from build123d import *

# Parameters (mm, degrees)
ESQUISSE1_W        = 176
ESQUISSE1_H        = 316
ESQUISSE1_W_2      = 70
ESQUISSE1_H_2      = 110
BOSS_EXTRU_1_DEPTH = 2
CONG_1_R           = 20


with BuildPart() as part:
    # Esquisse1 → Boss.-Extru.1 (new body)
    with BuildSketch(Plane.XY):
        with Locations((88, 158)):
            Rectangle(ESQUISSE1_W, ESQUISSE1_H)
        with Locations((131, 80)):
            Rectangle(ESQUISSE1_W_2, ESQUISSE1_H_2, mode=Mode.SUBTRACT)
    extrude(amount=BOSS_EXTRU_1_DEPTH)

    # Congé1
    cong_1_edges = [part.edges().sort_by_distance(p)[0] for p in [
        (166, 25, 1),
        (166, 135, 1),
        (96, 135, 1),
        (96, 25, 1),
    ]]
    fillet(cong_1_edges, radius=CONG_1_R)


solid = part.part
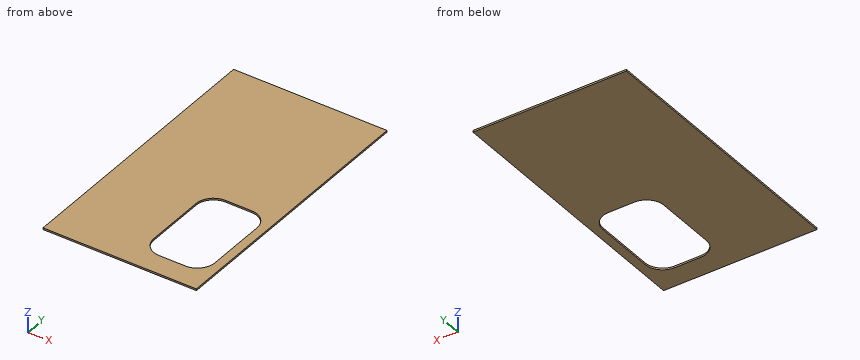
Input: part model. Units: mm. Frame: model coordinates. Coordinates: 2 decimals unless noted, no trailing zeros. Order: outer loops, then holes, each group sorted by start corner. A loop starts at its lowest first (then second) coordinate and runs counter-clockwise, first axis right, second up. Notation, with made-up numbers: M 40.25,59 L 69.25,59 A30 ccw 69.25,97 Z; hole C -36,1.5 d2. An arc over 180 degrees is marked long. Answer in a Markdown table with one row per item.
(1) Section query B-B, the plane z = 0.3. Output: boundary loops of the cut face in (x, y), plus the area to 3 significant figures.
Numbers:
| item | result |
|---|---|
| outline | M 0,0 L 176,0 L 176,316 L 0,316 Z; hole M 96,45 A20 ccw 116,25 L 146,25 A20 ccw 166,45 L 166,115 A20 ccw 146,135 L 116,135 A20 ccw 96,115 Z |
| area | 48,300 mm^2 |
(2) Material intervals for line 1 (X direction, y = 64.5, z = 0.95); line 2 (Y direction, x = 103, z = 1.9); line 3 (Y direction, x = 105.5, z = 0.4), sorted ascending. Write a range as [from, to].
Numbers:
| item | result |
|---|---|
| line 1 | x = [0, 96], [166, 176] |
| line 2 | y = [0, 29.8], [130.2, 316] |
| line 3 | y = [0, 27.98], [132.02, 316] |
(3) Section query C-C, the plane y = 104.5. Output: boundary loops of the cut face in (x, z).
Numbers:
| item | result |
|---|---|
| outline | M 0,0 L 96,0 L 96,2 L 0,2 Z; M 166,0 L 176,0 L 176,2 L 166,2 Z |
(4) Section query A-A, the plane y = 29. Output: boundary loops of the cut face in (x, z), plus the area to 3 significant figures.
Numbers:
| item | result |
|---|---|
| outline | M 0,0 L 104,0 L 104,2 L 0,2 Z; M 158,0 L 176,0 L 176,2 L 158,2 Z |
| area | 244 mm^2 |
